from build123d import *

# Parameters (mm, degrees)
F0_R      = 13.50645
F1_DEPTH  = 2.54
F2_W      = 27.0256
F2_H      = 76.2
F3_DEPTH  = 2.54
F4_R      = 1.778
F5_DEPTH  = 2.541
F7_DEPTH  = 26.9875
F9_DEPTH  = 26.9875
F10_R     = 60.96
F10_W     = 26.9875
F10_H     = 2.1313130632
F11_DEPTH = 50.8
F12_R     = 56.5455680067
F13_DEPTH = 116.7461731313
F15_DEPTH = 50.801
F17_DEPTH = 50.8
F19_DEPTH = 25.4
F20_DEPTH = 26.9875
F21_DEPTH = 25.4


# Not quite as in the source:
# - a feature names something its author has since deleted; it is built from what else it names


with BuildPart() as f1:
    # F0 (on Top) → F1 (new body)
    with BuildSketch(Plane.XY):
        with Locations((0, 38.9145108197)):
            Circle(F0_R)
    extrude(amount=F1_DEPTH)

    # F2 (on Top) → F3 (join)
    with BuildSketch(Plane.XY):
        with Locations((0.0679422232, -0.4738955459)):
            Rectangle(F2_W, F2_H)
    extrude(amount=F3_DEPTH)

    # F4 (on Top) → F5 (cut, through all)
    with BuildSketch(Plane.XY):
        with Locations((-8.2149387259, 41.2970071224)):
            Circle(F4_R)
        with Locations((0, 48.1029608197)):
            Circle(F4_R)
        with Locations((0, 33.1169608197)):
            Circle(F4_R)
        with Locations((8.2149387259, 41.2970071224)):
            Circle(F4_R)
    extrude(amount=F5_DEPTH, mode=Mode.SUBTRACT)

    # F6 (on face) → F7 (join)
    with BuildSketch(Plane.YZ.offset(13.5807422232)):
        Polygon((-136.5347272621, 116.7451731313), (-38.5738955459, 0), (-38.5738955459, 2.54), (-134.4034141989, 116.7451731313), align=None)
    extrude(amount=-F7_DEPTH)

    # F8 (on face) → F9 (join)
    with BuildSketch(Plane(origin=(-13.4067577768, 0, 0), x_dir=(0, -1, 0), z_dir=(-1, 0, 0))):
        Polygon((38.5738955459, 2.54), (49.0018958172, 14.9676067869), (16.4343814087, 2.54), align=None)
    extrude(amount=-F9_DEPTH)


with BuildPart() as f11:
    # F10 (on face) → F11 (new body)
    with BuildSketch(Plane.XY.offset(116.7451731313)):
        with Locations((0, -175.3809303045)):
            Circle(F10_R)
        with Locations((0.0869922232, -135.4690707305)):
            Rectangle(F10_W, F10_H, mode=Mode.SUBTRACT)
    extrude(amount=-F11_DEPTH)

    # F12 (on face) → F13 (cut, through all)
    with BuildSketch(Plane.XY.offset(116.7451731313)):
        with Locations((-8.7670916691, -175.4986345768)):
            Circle(F12_R)
    extrude(amount=-F13_DEPTH, mode=Mode.SUBTRACT)

    # F14 (on face) → F15 (cut, through all)
    with BuildSketch(Plane(origin=(0, 0, 65.9451731313), x_dir=(1, 0, 0), z_dir=(0, 0, -1))):
        with BuildLine():
            ThreePointArc((-34.6411562373, 125.2200701191), (-26.8424040995, 120.6487921939), (-18.4533903647, 117.2810681356))
            Line((-18.4533903647, 117.2810681356), (-18.4533903647, 119.7888788891))
            ThreePointArc((-18.4533903647, 119.7888788891), (-26.7534564605, 121.8899417854), (-34.6411562373, 125.2200701191))
        make_face()
    extrude(amount=-F15_DEPTH, mode=Mode.SUBTRACT)

    # F16 (on face) → F17 (cut)
    with BuildSketch(Plane(origin=(0, 0, 65.9451731313), x_dir=(1, 0, 0), z_dir=(0, 0, -1))):
        with BuildLine():
            Line((-12.9449410231, 231.889651911), (-12.9449410231, 234.9506382265))
            ThreePointArc((-12.9449410231, 234.9506382265), (-23.5006925786, 231.6289440324), (-33.2820246218, 226.4537061942))
            ThreePointArc((-33.2820246218, 226.4537061942), (-23.3686777331, 230.1264200492), (-12.9449410231, 231.889651911))
        make_face()
    extrude(amount=-F17_DEPTH, mode=Mode.SUBTRACT)


with BuildPart() as f19:
    # F18 (on face) → F19 (new body)
    with BuildSketch(Plane(origin=(-13.4067577768, 0, 0), x_dir=(0, -1, 0), z_dir=(-1, 0, 0))):
        Polygon((116.024311172, 92.3018110703), (105.3223571677, 79.5477189379), (117.2810681356, 79.5477189379), align=None)
    extrude(amount=F19_DEPTH)


with BuildPart() as f20:
    # F18 (on face) → F20 (new body)
    with BuildSketch(Plane(origin=(-13.4067577768, 0, 0), x_dir=(0, -1, 0), z_dir=(-1, 0, 0))):
        Polygon((116.024311172, 92.3018110703), (105.3223571677, 79.5477189379), (117.2810681356, 79.5477189379), align=None)
    extrude(amount=-F20_DEPTH)


with BuildPart() as f21_tool:
    # F21 (cut): a face of the model
    f21_faces = [f19.part.faces().sort_by_distance(p)[0] for p in [
        (-38.8067577768, -112.8759121584, 83.7990829821),
    ]]
    extrude(f21_faces, amount=-F21_DEPTH)


with BuildPart() as f11_1:
    add(f11.part)

    # F21: cut by f21_tool
    add(f21_tool.part, mode=Mode.SUBTRACT)


with BuildPart() as f19_1:
    add(f19.part)

    # F21: cut by f21_tool
    add(f21_tool.part, mode=Mode.SUBTRACT)


solid = f1.part
Source: CAD feature listing. Evaluate the final solid. Frame: model axes, mm. Give positions to 0.01 mm unless a question says otherwise; leave off trailing zeros. Order: outer loops, then holes, each group sorted by start corner. A loop starts at its lowest first (then second) coordinate and runs counter-clockwise, first axis right, second up. Notation, with made-up numbers: (-23.75, -22.75) -> (-16.75, -22.75) arc R25 ccw to (-16.75, 5.25) -> close; hole circle Ø1 at (-29.5, -28). An arc over 180 degrees is marked (long way). Write item = value, one per line.
Q1. Cut plane C-C, the plane z = 84.5. Output: boundary loops of the cut face in (x, y).
Data:
outline = (-13.41, -109.48) -> (13.58, -109.48) -> (13.58, -107.35) -> (-13.41, -107.35) -> close
Q2. Cut plane B-B, the plane x = -4.5. Output: boundary loops of the cut face in (y, z), and give its area (3 significant figures).
Data:
outline = (-136.53, 116.75) -> (-38.57, 0) -> (51.65, 0) -> (51.65, 2.54) -> (-16.43, 2.54) -> (-49, 14.97) -> (-134.4, 116.75) -> close
area = 613 mm^2
Q3. Pin query (flat end, axial travel): pin 1 (2 mm diameter, centred on x = -6, z = 46.5, fed in from -Y); pin 2 (2 mm diameter, centred on x = -5, y = -51.5, fed in from -Z); pin 3 (8 mm diameter, centred on x = -3.5, y = 1, fed in from +Z). Return the tip coordinate at first contact, or that it passes through.
Data:
pin_1 = -78.43
pin_2 = 14.21
pin_3 = 2.54
Q4. Material intervals for line 1 (Z direction, x = 5.5, y = 6); line 2 (Y direction, x = 1, z = 46); line 3 (Y direction, x = -1, z = 17.5), sorted ascending. Write a range as from..to.
Data:
line_1 = 0..2.54
line_2 = -77.17..-75.04
line_3 = -53.26..-51.13
Q5. Cut plane A-A, the plane y = 12. Output: boundary loops of the cut face in (x, z), and give its area (3 significant figures).
Data:
outline = (-13.44, 0) -> (13.58, 0) -> (13.58, 2.54) -> (-13.44, 2.54) -> close
area = 68.6 mm^2
Q6. Pull-direction query (X, two-part tool) for faces 1 (the face through (9, 39.7, 1.3)), 2 (the face through (-13.407, -76, 46)), 3 (the face through (0.28, -88.24, 59.19)), 4 (the face through (-0.385, 31.381, 1.252)); classes: released by +X, released by -X, zero draft, split by the parting line, or undercut.
Data:
face_1 = undercut
face_2 = released by -X
face_3 = zero draft
face_4 = undercut
